Input: part model. Units: mm. Frame: model coordinates. A direction names the side the tool comes from. Round coordinates to 2 decimals unless told otherwise and drop trailing zeros. Write each loop counter-clockwise with the first axis right and the second up, starting at its lowest first coordinate (ties: lowest second). Pieces come first, ordered by that corner, then holes. Notation, with made-up numbers: M 46,-5.5 L 57,-5.5 A18 ccw 57,13.5 Z; hole C 2,10.25 d7. An arc over 180 degrees is marked long. Answer as CSV lines item,"result". Start each with the question number.
Autodesk Inventor part; units mm, degrees
ref_plane "YZ Plane" through (0, 0, 0) normal (1, 0, 0) x (0, 1, 0)
ref_plane "XZ Plane" through (0, 0, 0) normal (0, 1, 0) x (-1, 0, 0)
ref_plane "XY Plane" through (0, 0, 0) normal (0, 0, 1) x (1, 0, 0)
sketch "Sketch1" plane through (0, 0, 0) normal (0, 0, 1) x (1, 0, 0)
  line L0 (0, 0) -> (46.99, 0)
  line L1 (46.99, 0) -> (46.99, 9.525)
  line L2 (46.99, 9.525) -> (44.8564, 9.525)
  line L3 (44.8564, 9.525) -> (43.0233, 6.35)
  line L4 (43.0233, 6.35) -> (0, 6.35)
  line L5 (0, 6.35) -> (0, 0)
  dimension "d0" = 44.8564
  dimension "d2" = 9.525
  dimension "d3" = 60
  dimension "d4" = 46.99
  dimension "d7" = 3.175
revolve "Revolution1" add sketch "Sketch1" angle 360 about axis through (0, 6.35, 0) along (0, -1, 0)
fillet "Fillet1" radius 1.5875 2 edges at (-44.8564, 9.525, 0) (-43.0233, 6.35, 0)
sketch "Sketch2" plane through (0, 6.35, 0) normal (0, 1, 0) x (1, 0, 0)
  circle A0 centre (0, 0) radius 41.275
  line L0 (-19.05, 36.6159) -> (-19.05, -36.6159)
  line L1 (19.05, -36.6159) -> (19.05, 36.6159)
  dimension "d8" = 82.55
  dimension "d9" = 38.1
extrude "Extrusion1" cut sketch "Sketch2" against normal through all contours L1 A0 L0
sketch "Sketch3" plane through (0, 6.35, 0) normal (0, 1, 0) x (1, 0, 0)
  line L0 (0, 0) -> (-30.48, 0) construction
  line L1 (0, 0) -> (30.48, 0) construction
  dimension "d12" = 60.96
hole "Hole1" at (-30.48, 6.35, 0) at (30.48, 6.35, 0) direction (0, -1, 0) diameter 8.89 end through all counterbore diameter 12.954 counterbore depth 4.7752
sketch "Sketch4" plane through (0, 0, 0) normal (0, -1, 0) x (1, 0, 0)
  line L0 (25.4, -19.05) -> (-25.4, -19.05) construction
  line L1 (-25.4, -19.05) -> (-25.4, 19.05) construction
  line L2 (-25.4, 19.05) -> (25.4, 19.05) construction
  line L3 (25.4, 19.05) -> (25.4, -19.05) construction
  line L4 (25.4, -19.05) -> (-25.4, 19.05) construction
  line L5 (25.4, 19.05) -> (-25.4, -19.05) construction
  point P0 (0, 0)
  point P1 (0, 0)
  dimension "d20" = 50.8
  dimension "d21" = 38.1
hole "Hole2" at (25.4, 0, -19.05) at (-25.4, 0, -19.05) at (-25.4, 0, 19.05) at (25.4, 0, 19.05) direction (0, 1, 0) diameter 5.207 end through all counterbore diameter 8.7313 counterbore depth 4.826
fillet "Fillet2" radius 3.175 4 edges at (19.05, 3.175, -36.6159) (19.05, 3.175, 36.6159) (-19.05, 3.175, 36.6159) (-19.05, 3.175, -36.6159)
properties part number "CarriageCap" material "ABS Plastic"
Item 1: Pin query (flat end, axial travel): pin 1 Ø1.5 at (y, z) = (7, 20) entering from -X; pin 2 Ø2 at (x, z) = (-21.5, 37.5) entering from +Y; pin 3 Ø7 at (x, z) = (-25.4, 19.05) entering from +Y. Return the tip coordinate at first contact, or that it passes through.
Item 2: Cut plane C-C, the plane y = 3. Return loops of the section in (x, z) (3 decimals), plus the area to 3 significant figures.
Item 3: Cut plane B-B, the plane z = 0. Give the number of separate pieces and of enclosed holes in the cut face, plus the area to 3 significant figures.
Item 4: Access query for faces 1 (the face through (-18.56, 3.13, -36.33)), 2 (the face through (-26, 1.575, -2)), 3 (the face through (20, 0, 1)), 4 (the face through (29.66, 2.45, -18.1)). Directions: +Z, -Z, +X, -X, +Y, -Y. A direction counts if a zero-diameter tool reaches every point of the face in a straight line with its end or side. Return the directions, or none.
Item 5: Draft query along Z for faces 5 (the face through (45, 9.525, -10)), 6 (the face through (25, 4.826, -22)), 7 (the face through (28.06, 2.45, 22.51)). Return one class per face: +Z half, -Z half, draft (parallel to the pull), parting line (faces both ways), or undercut.
Item 6: Line query: line 1 (X direction, y = 5.6, z = 19.05); line 2 (X direction, y = 3, z = 21.5); line 3 (Y direction, x = -15.5, z = -39). Output: solid intervals per line, ascending. Write a range as [from, to].
Results list:
1,pin 1,"x = -42.87"
1,pin 2,"y = 8.43"
1,pin 3,"y = 6.35"
2,outline,"C 0,0 d93.98; hole C -30.48,0 d12.954; hole C -25.4,-19.05 d8.731; hole C -25.4,19.05 d8.731; hole M -19.05,-34.635 A3.175 ccw -17.198,-37.521 A41.275 ccw 17.198,-37.521 A3.175 ccw 19.05,-34.635 L 19.05,34.635 A3.175 ccw 17.198,37.521 A41.275 ccw -17.198,37.521 A3.175 ccw -19.05,34.635 Z; hole C 25.4,-19.05 d8.731; hole C 25.4,19.05 d8.731; hole C 30.48,0 d12.954"
2,area,"3,410 mm²"
3,separate pieces,"4"
3,enclosed holes,"0"
3,area,"222 mm²"
4,face 1,"+Y, -Y"
4,face 2,"+Y"
4,face 3,"+Z, -Z, +X, -X, -Y"
4,face 4,"-Y"
5,face 5,"draft"
5,face 6,"undercut"
5,face 7,"undercut"
6,line 1,"[-42.96, -28], [-22.8, -19.05], [19.05, 22.8], [28, 42.96]"
6,line 2,"[-41.78, -29.01], [-21.79, -19.05], [19.05, 21.79], [29.01, 41.78]"
6,line 3,"[0, 6.35]"
